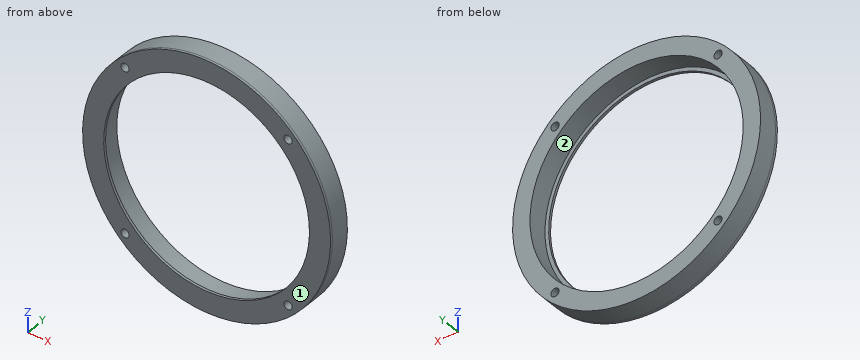
from build123d import *

# Parameters (mm, degrees)
SKETCH_2_R         = 50
SKETCH_2_R_2       = 43
EXTRUDE_1_DEPTH    = 8
EXTRUDE_START      = 1
SKETCH_3_R         = 50
SKETCH_3_R_2       = 41.5
EXTRUDE_2_DEPTH    = 1
HOLE_WIZARD_M4_1_D = 3.3


with BuildPart() as part:
    # 草图2 → 凸台-拉伸1 (new body)
    with BuildSketch(Plane(origin=(0, 0, 0), x_dir=(1, 0, 0), z_dir=(0, 1, 0))):
        with Locations(Location((0, 0, 0), (0, 0, 270))):
            Circle(SKETCH_2_R)
        with Locations(Location((0, 0, 0), (0, 0, 270))):
            Circle(SKETCH_2_R_2, mode=Mode.SUBTRACT)
    extrude(amount=EXTRUDE_1_DEPTH)

    # 草图3 → 凸台-拉伸2 (add)
    with BuildSketch(Plane.XZ.offset(EXTRUDE_START)):
        with Locations(Location((0, 0, 0), (0, 0, 270))):
            Circle(SKETCH_3_R)
        with Locations(Location((0, 0, 0), (0, 0, 270))):
            Circle(SKETCH_3_R_2, mode=Mode.SUBTRACT)
    extrude(amount=-EXTRUDE_2_DEPTH)

    # M4 螺纹孔1 (through all)
    with Locations(Plane(origin=(0, 8, 0), x_dir=(1, 0, 0), z_dir=(0, 1, 0))):
        with Locations((-32.880465325, 32.880465325), (-32.880465325, -32.880465325), (32.880465325, -32.880465325), (32.880465325, 32.880465325)):
            Hole(HOLE_WIZARD_M4_1_D / 2)


solid = part.part
Source: CAD feature listing. Evaluate the final solid. Frame: model axes, mm. Face numbers are marked on the shaded views. Round coordinates to 2 decimals unless told otherwise and drop trailing zeros. Loops run counter-clockwise (first coordinate to the right, second up) from the corner with the lowest first, then second, coordinate; pieces in that order, holes last. Notation, with made-up numbers: (37, 82) - (79, 82) arc R15 ccw to (79, 108) - close; hole circle Ø8 at (59, 25.5). An arc over 180 degrees is marked (long way). Write item = value, one per line. Start each with the question number.
Item 1: Section query C-C on y = 1.75. Output: boundary loops of the cut face in (x, z).
Item 2: Section query B-B on x = 0. Output: boundary loops of the cut face in (y, z), plus the area to 3 significant figures.
Item 3: Section query A-A on z = 0. Output: boundary loops of the cut face in (x, y).
Item 4: Mould query, pull axis X, two halves, no side actions, for the marked faces 1 and 2. Classes: released by +X, released by -X, zero draft, split by the parting line, or undercut.
Item 5: Material intervals for line 1 (X direction, y = 4.75, z = -31.5); line 2 (X direction, y = 2.25, z = -32.5); line 3 (Z direction, x = -1, y = 4), sorted ascending.
Item 6: First-contact query: pin 1 Ø2 at (x, z) = (32.88, 32.88) entering from +Y; pin 2 Ø3 at (y, z) = (1.5, -33) entering from +X; pin 3 Ø1 at (x, y) = (-3, 4) entering from +Z; pin 4 Ø2 at (x, y) = (-13.5, 6.5) entering from +Z. Flat tips, straight axial feed; report the tip coordinate or a pass-through.
Results list:
q1.outline = circle Ø100 at (0, 0); hole circle Ø86 at (0, 0); hole circle Ø3.3 at (-32.88, -32.88); hole circle Ø3.3 at (-32.88, 32.88); hole circle Ø3.3 at (32.88, -32.88); hole circle Ø3.3 at (32.88, 32.88)
q2.outline = (-1, -50) - (8, -50) - (8, -43) - (0, -43) - (0, -41.5) - (-1, -41.5) - close; (-1, 41.5) - (0, 41.5) - (0, 43) - (8, 43) - (8, 50) - (-1, 50) - close
q2.area = 129 mm²
q3.outline = (-50, -1) - (-41.5, -1) - (-41.5, 0) - (-43, 0) - (-43, 8) - (-50, 8) - close; (41.5, -1) - (50, -1) - (50, 8) - (43, 8) - (43, 0) - (41.5, 0) - close
q4.face_1 = zero draft
q4.face_2 = undercut
q5.line_1 = -38.83 to -33.78, -31.98 to -29.27, 29.27 to 31.98, 33.78 to 38.83
q5.line_2 = -38 to -34.49, -31.27 to -28.16, 28.16 to 31.27, 34.49 to 38
q5.line_3 = -49.99 to -42.99, 42.99 to 49.99
q6.pin_1 = through
q6.pin_2 = 38.83
q6.pin_3 = 49.94
q6.pin_4 = 48.41
